from build123d import *

# Parameters (mm, degrees)
SKETCH1_R           = 3.915
BOSS_EXTRUDE1_DEPTH = 4


with BuildPart() as part:
    # Sketch1 → Boss-Extrude1 (new body)
    with BuildSketch(Plane(origin=(0, 0, 0), x_dir=(1, 0, 0), z_dir=(0, 1, 0))):
        with BuildLine():
            Line((112.296761578, 6.055177331), (112.296761578, 3.119444466))
            ThreePointArc((112.296761578, 3.119444466), (117.173733569, 1.869604275), (122.191807827, 2.276896615))
            ThreePointArc((122.191807827, 2.276896615), (127.614961562, 16.075321721), (142.200280719, 18.735321146))
            Line((142.200280719, 18.735321146), (141.13131283, 32.295700632))
            Line((141.13131283, 32.295700632), (106.296761578, 32.295700632))
            Line((106.296761578, 32.295700632), (106.296761578, 6.055177331))
            Line((106.296761578, 6.055177331), (112.296761578, 6.055177331))
        make_face()
        with Locations(Location((118.466761578, 17.055177331, 0), (0, 0, 270))):
            Circle(SKETCH1_R, mode=Mode.SUBTRACT)
    extrude(amount=BOSS_EXTRUDE1_DEPTH)


solid = part.part
Geometry: final body of the model. Coordinates: model frame, mm. A direction names the side the tool comes from. Give positions to 0.01 mm unless a question says otherwise; leave off trailing zeros. Write each loop counter-clockwise with the first axis right and the second up, starting at its lowest first coordinate (ties: lowest second). Pieces come first, ordered by that corner, then holes. Notation, with made-up numbers: (-21.5, 40.5) - (-2.5, 40.5) arc R20 ccw to (-2.5, 62.5) - close; hole circle Ø6 at (-12, 49.5). An arc over 180 degrees is marked (long way). Return JSON: item names as keys, results as strings. Group by question number.
1) Section D-D on x = 111.5. Return the cut outline in (y, z), plus the area to 3 significant figures.
2) Section C-C on y = 1.5. Return the cut outline in (x, z) (3 decimals).
3) Set-up query: faces 4 (the flat face through (109, 2, -6.055)), 5 (the flat face through (141.673, 1.972, -25.421)). Return all of +Z, -Z, +X, -X, +Y, -Y with unobstructed straight access to the full face (end or side cutting, diameter ignored); none if empty.
4) Section B-B on x = 118. Return the cut outline in (y, z), plus the area to 3 significant figures.
5) Mould query, pull axis X, two halves, no side actions, for faces 1 (the flat face through (120, 4, -21)), 2 (the cylindrical face through (121.8, 2, -15)), 3 (the flat face through (112.297, 2, -5)). Classes: released by +X, released by -X, zero draft, split by the parting line, or undercut.
6) Section A-A on z = -18. Return the cut outline in (x, y), plus the area to 3 significant figures.
7) Line query: line 1 (Z direction, x = 108.5, y = 2.6); line 2 (X direction, y = 3.5, z = -4); line 3 (Z direction, x = 115, y = 2.15). Output: solid intervals per line, ascending.
8) First-contact query: P1, Ø1.5, axis at y = 3, z = -12, coming from the +X side. Flat tip, straight axial feed; report the tip coordinate or a pass-through.
Filled in:
{
 "1": {"outline": "(0, -32.3) - (4, -32.3) - (4, -6.06) - (0, -6.06) - close", "area": "105 mm^2"},
 "2": {"outline": "(106.297, -32.296) - (141.131, -32.296) - (142.2, -18.735) arc R15.241 cw to (122.192, -2.277) arc R15.241 ccw to (112.297, -3.119) - (112.297, -6.055) - (106.297, -6.055) - close; hole circle Ø7.83 at (118.467, -17.055)"},
 "3": {"face 4": "+Z, -X, +Y, -Y", "face 5": "-Z, +X, +Y, -Y"},
 "4": {"outline": "(0, -32.3) - (4, -32.3) - (4, -20.94) - (0, -20.94) - close; (0, -13.17) - (4, -13.17) - (4, -1.82) - (0, -1.82) - close", "area": "90.8 mm^2"},
 "5": {"face 1": "zero draft", "face 2": "undercut", "face 3": "released by -X"},
 "6": {"outline": "(106.3, 0) - (114.67, 0) - (114.67, 4) - (106.3, 4) - close; (122.27, 0) - (130.61, 0) - (130.61, 4) - (122.27, 4) - close", "area": "66.9 mm^2"},
 "7": {"line 1": "z = -32.3 to -6.06", "line 2": "x = 112.3 to 122.06", "line 3": "z = -32.3 to -18.87, -15.24 to -2.21"},
 "8": {"P1": "stops at x = 124.61"}
}
